Input: part model. Units: mm. Frame: model coordinates. A direction names the side the tool comes from. Coordinates: 2 decimals unless noted, no trailing zeros. Loops run counter-clockwise (first coordinate to the right, second up) from the corner with the lowest first, then second, coordinate; pieces in that order, holes last.
(1) Set-up query: faces 5 (the face through (0, -2, 65)), 6 (the face through (-31.533, -2.535, 58.495)). Return all of +Z, -Z, +X, -X, +Y, -Y with unobstructed straight access to the full face (end or side cutting, diameter ignored); none if empty.
(2) Section A-A, the plane x = -12. Return loops of the section in (y, z), then the cut area to 3 significant figures.
(3) Section B-B, the plane z = -25. Return loops of the section in (x, y) (1 decimal).
(4) Line query: L1, parallel to Z at x = 10, y = -1.7; L2, parallel to X at y = -1.65, z = -6 (1 decimal); L3, parallel to X at y = -3.7, z = -57.5. Output: solid intervals per line, ascending.
(5) Mould query, pull axis X, two halves, no side actions, for faces 1 (the face through (-31.533, -2.535, -58.495)), 2 (the face through (0, -2, -65)), 3 (the face through (0, -2, -59.35)), 4 (the face through (-35.348, -2.535, 63.496)). Classes: released by +X, released by -X, zero draft, split by the parting line, or undercut.
```python
from build123d import *

# Parameters (mm, degrees)
F0_W     = 73.547
F0_H     = 130
F0_W_2   = 64.87
F0_H_2   = 118.7
F1_DEPTH = 5
F2_R     = 5
F3_R     = 3


with BuildPart() as f1:
    # F0 (on Front) → F1 (new body)
    with BuildSketch(Plane.XZ):
        Rectangle(F0_W, F0_H)
        Rectangle(F0_W_2, F0_H_2, mode=Mode.SUBTRACT)
    extrude(amount=F1_DEPTH)

    # F2
    f2_edges = [f1.edges().sort_by_distance(p)[0] for p in [
        (-36.7735, -2.5, 65),
        (36.7735, -2.5, 65),
        (36.7735, -2.5, -65),
        (-36.7735, -2.5, -65),
    ]]
    fillet(f2_edges, radius=F2_R)

    # F3
    f3_edges = [f1.edges().sort_by_distance(p)[0] for p in [
        (32.435, -2.5, 59.35),
        (32.435, -2.5, -59.35),
        (-32.435, -2.5, 59.35),
        (-32.435, -2.5, -59.35),
    ]]
    fillet(f3_edges, radius=F3_R)


solid = f1.part
```
Report:
1. face 5: +Z, +X, -X, +Y, -Y
1. face 6: +Y, -Y
2. outline: (-5, -65) - (0, -65) - (0, -59.35) - (-5, -59.35) - close; (-5, 59.35) - (0, 59.35) - (0, 65) - (-5, 65) - close
2. area: 56.5 mm2
3. outline: (-36.8, -5) - (-32.4, -5) - (-32.4, 0) - (-36.8, 0) - close; (32.4, -5) - (36.8, -5) - (36.8, 0) - (32.4, 0) - close
4. L1: z = -65 to -59.35, 59.35 to 65
4. L2: x = -36.8 to -32.4, 32.4 to 36.8
4. L3: x = -36.77 to -32.21, 32.21 to 36.77
5. face 1: undercut
5. face 2: zero draft
5. face 3: undercut
5. face 4: released by -X
